```python
from build123d import *

# Parameters (mm, degrees)
BOSS_EXTRUDE1_DEPTH     = 3.7338
BOSS_EXTRUDE2_DEPTH     = 3.7338
CUT_EXTRUDE1_DEPTH      = 197.398400929
FILLET7_R               = 9.525
FILLET8_R               = 3.175
F_8_32_TAPPED_HOLE2_D   = 4.1656
FILLET3_RADIUS          = 1.8669
FILLET3_LENGTH          = 19.05
FILLET4_RADIUS          = 1.8669
FILLET4_LENGTH          = 19.05
FILLET5_RADIUS          = 1.8669
FILLET5_LENGTH          = 19.05
FILLET6_START           = -20
FILLET6_DEPTH           = 22
CUT_EXTRUDE2_START      = -5
CUT_EXTRUDE2_OUTLINE_R  = 2.2479
CUT_EXTRUDE2_DEPTH      = 6
CUT_EXTRUDE3_DEPTH      = 196.819265209
SKETCH15_W              = 94.065777876
SKETCH15_H              = 7.9375
CUT_EXTRUDE4_DEPTH      = 196.819265209
SKETCH16_W              = 20.234222124
SKETCH16_H              = 6.35
CUT_EXTRUDE5_DEPTH      = 196.819265209
CUT_EXTRUDE6_DEPTH      = 196.819265209
CUT_EXTRUDE6_DEPTH_BACK = 196.819265209
SKETCH17_W              = 3.175
SKETCH17_H              = 3.175


with BuildPart() as part:
    # Sketch1 → Boss-Extrude1 (new body)
    with BuildSketch(Plane.XY):
        Polygon((0, 0), (9.525, 0), (9.525, -19.05), (20.6375, -19.05), (20.6375, 0), (46.0375, 0), (46.0375, -19.05), (180.975, -19.05), (180.975, 0), (-16.893133293, 76.2), align=None)
    extrude(amount=BOSS_EXTRUDE1_DEPTH)

    # Sketch7 → Boss-Extrude2 (add)
    with BuildSketch(Plane.XY.offset(3.7338)):
        Polygon((-161.613635382, -74.129081959), (-0.247657199, 1.117109433), (-16.893133293, 76.2), (-166.605179671, -63.424680687), align=None)
    extrude(amount=-BOSS_EXTRUDE2_DEPTH)

    # Sketch8 → Cut-Extrude1 (cut, through all)
    with BuildSketch(Plane.XY.offset(3.7338)):
        Polygon((2.518832326, 10.642109433), (126.836493994, 10.642109433), (-9.085614858, 62.98638803), align=None)
        Polygon((-18.542737866, 61.637057548), (-138.674453357, -50.400369109), (-7.28718114, 10.86652211), align=None)
    extrude(amount=-CUT_EXTRUDE1_DEPTH, mode=Mode.SUBTRACT)

    # Fillet7
    fillet7_edges = [part.edges().sort_by_distance(p)[0] for p in [
        (-16.893133293, 76.2, 1.8669),
    ]]
    fillet(fillet7_edges, radius=FILLET7_R)

    # Fillet8
    fillet8_edges = [part.edges().sort_by_distance(p)[0] for p in [
        (-9.085614858, 62.98638803, 1.8669),
        (126.836493994, 10.642109433, 1.8669),
        (2.518832326, 10.642109433, 1.8669),
        (-7.28718114, 10.86652211, 1.8669),
        (-138.674453357, -50.400369109, 1.8669),
        (-18.542737866, 61.637057548, 1.8669),
    ]]
    fillet(fillet8_edges, radius=FILLET8_R)

    # #8-32 Tapped Hole2 (through all)
    with Locations(Plane.XY.offset(3.7338)):
        with Locations((15.08125, -11.1125), (58.7375, -11.1125), (168.275, -7.9375)):
            Hole(F_8_32_TAPPED_HOLE2_D / 2)

    # Fillet3: full round fillet: the end face becomes a half cylinder, R = half its width
    fillet3_face = Plane((9.525, -9.525, 1.8669), x_dir=(0, 1, 0), z_dir=(-1, 0, 0))  # on the end face: x along it, z out of the body
    fillet3_slab = fillet3_face.offset(-FILLET3_RADIUS / 2) * Box(FILLET3_LENGTH, 2 * FILLET3_RADIUS, FILLET3_RADIUS, mode=Mode.PRIVATE)  # the body's end, R deep
    fillet3_round = Plane((11.3919, -9.525, 1.8669), x_dir=(-1, 0, 0), z_dir=(0, 1, 0)) * Cylinder(FILLET3_RADIUS, FILLET3_LENGTH, mode=Mode.PRIVATE)  # its axis R under the face
    add(fillet3_slab - fillet3_round, mode=Mode.SUBTRACT)

    # Fillet4: full round fillet: the end face becomes a half cylinder, R = half its width
    fillet4_face = Plane((20.6375, -9.525, 1.8669), x_dir=(0, 1, 0), z_dir=(1, 0, 0))  # on the end face: x along it, z out of the body
    fillet4_slab = fillet4_face.offset(-FILLET4_RADIUS / 2) * Box(FILLET4_LENGTH, 2 * FILLET4_RADIUS, FILLET4_RADIUS, mode=Mode.PRIVATE)  # the body's end, R deep
    fillet4_round = Plane((18.7706, -9.525, 1.8669), x_dir=(1, 0, 0), z_dir=(0, 1, 0)) * Cylinder(FILLET4_RADIUS, FILLET4_LENGTH, mode=Mode.PRIVATE)  # its axis R under the face
    add(fillet4_slab - fillet4_round, mode=Mode.SUBTRACT)

    # Fillet5: full round fillet: the end face becomes a half cylinder, R = half its width
    fillet5_face = Plane((46.0375, -9.525, 1.8669), x_dir=(0, -1, 0), z_dir=(-1, 0, 0))  # on the end face: x along it, z out of the body
    fillet5_slab = fillet5_face.offset(-FILLET5_RADIUS / 2) * Box(FILLET5_LENGTH, 2 * FILLET5_RADIUS, FILLET5_RADIUS, mode=Mode.PRIVATE)  # the body's end, R deep
    fillet5_round = Plane((47.9044, -9.525, 1.8669), x_dir=(-1, 0, 0), z_dir=(0, -1, 0)) * Cylinder(FILLET5_RADIUS, FILLET5_LENGTH, mode=Mode.PRIVATE)  # its axis R under the face
    add(fillet5_slab - fillet5_round, mode=Mode.SUBTRACT)

    # Fillet6: read off the stored shape, not the designer's step
    # Fillet6 outline → Fillet6 (cut)
    with BuildSketch(Plane(origin=(0, 0, 0), x_dir=(1, 0, 0), z_dir=(0, 1, 0)).offset(FILLET6_START)):
        with BuildLine():
            ThreePointArc((179.1081, 0), (180.42819765, -0.54680235), (180.975, -1.8669))
            Line((180.975, -1.8669), (180.975, 0))
            Line((180.975, 0), (179.1081, 0))
        make_face()
        with BuildLine():
            ThreePointArc((180.975, -1.8669), (180.42819765, -3.18699765), (179.1081, -3.7338))
            Line((179.1081, -3.7338), (180.975, -3.7338))
            Line((180.975, -3.7338), (180.975, -1.8669))
        make_face()
    extrude(amount=FILLET6_DEPTH, mode=Mode.SUBTRACT)

    # Cut-Extrude2: read off the stored shape, not the designer's step
    # Cut-Extrude2 outline → Cut-Extrude2 (cut)
    with BuildSketch(Plane.XY.offset(3.7338).offset(CUT_EXTRUDE2_START)):
        with Locations((-124.299564913, -48.97170394)):
            Circle(CUT_EXTRUDE2_OUTLINE_R)
        with Locations((-158.829891599, -65.073459713)):
            Circle(CUT_EXTRUDE2_OUTLINE_R)
        Polygon((-0.247657199, 1.117109433), (0, 0), (0, 1.232593882), align=None)
    extrude(amount=CUT_EXTRUDE2_DEPTH, mode=Mode.SUBTRACT)

    # Sketch14 → Cut-Extrude3 (cut, through all)
    with BuildSketch(Plane.XY.offset(3.7338)):
        with BuildLine():
            Line((71.4375, -6.35), (155.978277876, -6.35))
            ThreePointArc((155.978277876, -6.35), (160.740777876, -11.1125), (155.978277876, -15.875))
            Line((155.978277876, -15.875), (71.4375, -15.875))
            ThreePointArc((71.4375, -15.875), (66.675, -11.1125), (71.4375, -6.35))
        make_face()
    extrude(amount=-CUT_EXTRUDE3_DEPTH, mode=Mode.SUBTRACT)

    # Sketch15 → Cut-Extrude4 (cut, through all)
    with BuildSketch(Plane.XY.offset(3.7338)):
        with Locations((113.707888938, -15.08125)):
            Rectangle(SKETCH15_W, SKETCH15_H)
    extrude(amount=-CUT_EXTRUDE4_DEPTH, mode=Mode.SUBTRACT)

    # Sketch16 → Cut-Extrude5 (cut, through all)
    with BuildSketch(Plane.XY.offset(3.7338)):
        with Locations((170.857888938, -15.875)):
            Rectangle(SKETCH16_W, SKETCH16_H)
    extrude(amount=-CUT_EXTRUDE5_DEPTH, mode=Mode.SUBTRACT)

    # Sketch17 → Cut-Extrude6 (cut, two sides: drawn at the far end of the back side and taken through both)
    with BuildSketch(Plane.XY.offset(3.7338).offset(-CUT_EXTRUDE6_DEPTH_BACK)):
        with Locations((19.05, -17.4625)):
            Rectangle(SKETCH17_W, SKETCH17_H)
    extrude(amount=CUT_EXTRUDE6_DEPTH + CUT_EXTRUDE6_DEPTH_BACK, mode=Mode.SUBTRACT)


solid = part.part
```
Could you check a few things on this model? Use its own coordinates, in mm. A direction names the side the tool comes from. Round coordinates to 2 decimals unless told otherwise and drop trailing zeros. Loops run counter-clockwise (first coordinate to the right, second up) from the corner with the lowest first, then second, coordinate; pieces in that order, holes last.
Q1. I want a section at A-A (x = 37). Write out the boundary of the cut face in (y, z), and give its area (3 significant figures).
Q2. I want a section at D-D (x = -135). Write out the boundary of the cut face in (y, z).
Q3. Please list where these lines run through material, in increasing order: L1, parallel to X at y = -18, z = 1.75 (1 decimal); L2, parallel to Y at x = 108, z = 1.4; L3, parallel to Y at x = 42, z = 0.85.
Q4. I want a section at C-C (z = 0.7). Give the number of separate pieces and of enclosed holes in the cut face, and give its area (3 significant figures).
Q5. For P1, Ø1, axis at x = -125, z = 1, coming from the -Y side; P2, Ø1.9, axis at x = 33.5, z = 2, coming from the -Y side; P3, Ø1, axis at y = 0.5, z = 1, coming from the -X side, each with a flat end and sliding along its axis, tell me the tip position at first contact or that it passes through.
Q6. Thinking about a two-plate mould opening in Y: for faces 1 (the flat face through (54.5, 38.5, 1.9)), 2 (the flat face through (86.2, 36.5, 1.8)), 3 (the flat face through (5, 1, 0)), which applies, pulls with the +Y half, pulls with the -Y half, needs draft (parallel to the pull), parting line crosses it, or undercut?
Q7. I want a section at B-B (y = 41.5). Write out the boundary of the cut face in (x, z), and give its area (3 significant figures).
Q8. On a 3-axis mill with a long thin cutter (end or side, diameter ignored), from which of +Z, -Z, +X, -X, +Y, -Y can I reach the whole of each face in a straight line? I mean faces 4 (the flat face through (-72.6, 11.22, 1.89)), 5 (the flat face through (5, 1, 3.734)). Say none if no direction works.
Answer below:
1. outline: (0, 0) - (10.64, 0) - (10.64, 3.73) - (0, 3.73) - close; (45.24, 0) - (55.45, 0) - (55.45, 3.73) - (45.24, 3.73) - close
1. area: 77.8 mm2
2. outline: (-61.72, 0) - (-33.95, 0) - (-33.95, 3.73) - (-61.72, 3.73) - close
3. L1: x = -117.9 to -103.9, -69.2 to -41.2, 9.5 to 17.5, 46 to 66.7
3. L2: y = -6.35 to 10.64, 17.9 to 28.1
3. L3: y = 0 to 10.64, 43.31 to 53.52
4. separate pieces: 1
4. enclosed holes: 7
4. area: 9,260 mm2
5. P1: stops at y = -57.29
5. P2: stops at y = 0
5. P3: stops at x = -98.6
6. face 1: undercut
6. face 2: pulls with the +Y half
6. face 3: needs draft
7. outline: (-54.1, 0) - (-40.13, 0) - (-40.13, 3.73) - (-54.1, 3.73) - close; (-14.08, 0) - (-4.32, 0) - (-4.32, 3.73) - (-14.08, 3.73) - close; (46.71, 0) - (73.21, 0) - (73.21, 3.73) - (46.71, 3.73) - close
7. area: 188 mm2
8. face 4: +Z, -Z
8. face 5: +Z, +X, -X, +Y, -Y
